from build123d import *

# Parameters (mm, degrees)
SKETCH_1_W                = 55
SKETCH_1_H                = 55
EXTRUDE_1_DEPTH           = 51
CUT_EXTRUDE_1_DEPTH       = 110.162722575
CHAMFER_1_SIZE            = 19.3
CUT_EXTRUDE_START         = -11
SKETCH_11_W               = 55
SKETCH_11_H               = 45
CUT_EXTRUDE_2_DEPTH       = 69.888985474
CUT_EXTRUDE_START_2       = 11
SKETCH_12_W               = 55
SKETCH_12_H               = 45
CUT_EXTRUDE_3_DEPTH       = 69.888985474
HOLE_WIZARD_M4_1_D        = 3.3
HOLE_WIZARD_M4_2_D        = 3.3
HOLE_WIZARD_1_D           = 6.6
HOLE_WIZARD_1_CBORE_D     = 11
HOLE_WIZARD_1_CBORE_DEPTH = 8
CUT_EXTRUDE_5_DEPTH       = 73.754724932
CUT_EXTRUDE_6_DEPTH       = 73.754724932
CHAMFER_2_SIZE            = 12
CUT_EXTRUDE_7_DEPTH       = 70.003623093


with BuildPart() as part:
    # 草图1 → 凸台-拉伸1 (new, symmetric)
    with BuildSketch(Plane.XY):
        Rectangle(SKETCH_1_W, SKETCH_1_H)
    extrude(amount=EXTRUDE_1_DEPTH, both=True)

    # 草图2 → 切除-拉伸1 (cut, through all)
    with BuildSketch(Plane.XY.offset(51)):
        Polygon((-27.5, -27.5), (16.5, -27.5), (-27.5, 16.5), align=None)
    extrude(amount=-CUT_EXTRUDE_1_DEPTH, mode=Mode.SUBTRACT)

    # 倒角1
    chamfer_1_edges = [part.edges().sort_by_distance(p)[0] for p in [
        (27.5, 27.5, 0),
    ]]
    chamfer(chamfer_1_edges, length=CHAMFER_1_SIZE)

    # 草图11 → 切除-拉伸2 (cut, through all)
    with BuildSketch(Plane.YZ.offset(27.5).offset(CUT_EXTRUDE_START)):
        with Locations((0, -28.5)):
            Rectangle(SKETCH_11_W, SKETCH_11_H)
    extrude(amount=-CUT_EXTRUDE_2_DEPTH, mode=Mode.SUBTRACT)

    # 草图12 → 切除-拉伸3 (cut, through all)
    with BuildSketch(Plane.XZ.offset(-27.5).offset(CUT_EXTRUDE_START_2)):
        with Locations((0, 28.5)):
            Rectangle(SKETCH_12_W, SKETCH_12_H)
    extrude(amount=CUT_EXTRUDE_3_DEPTH, mode=Mode.SUBTRACT)

    # M4 螺纹孔1 (through all)
    with Locations(Plane(origin=(16.5, -23.392318354, -4.126238011), x_dir=(0, 1, 0), z_dir=(-1, 0, 0))):
        with Locations((33.892318354, 26.873761989), (8.392318354, 41.596193853), (8.392318354, 12.151330125)):
            Hole(HOLE_WIZARD_M4_1_D / 2)

    # M4 螺纹孔2 (through all)
    with Locations(Plane(origin=(-3.776378322, 16.5, -11.360569787), x_dir=(-1, 0, 0), z_dir=(0, -1, 0))):
        with Locations((-14.276378322, -42.360569787), (11.223621678, -57.083001652), (11.223621678, -27.638137923)):
            Hole(HOLE_WIZARD_M4_2_D / 2)

    # 打孔尺寸根据内六角圆柱头螺钉的类型1 (through all)
    with Locations(Plane(origin=(-5.5, -5.5, 0), x_dir=(-0.7071067811865475, 0.7071067811865477, 0), z_dir=(-0.7071067811865477, -0.7071067811865475, 0))):
        with Locations((6.5, 0), (-6.5, 0)):
            CounterBoreHole(HOLE_WIZARD_1_D / 2, HOLE_WIZARD_1_CBORE_D / 2, HOLE_WIZARD_1_CBORE_DEPTH)

    # 草图22 → 切除-拉伸5 (cut, through all)
    with BuildSketch(Plane.XZ.offset(-16.5)):
        Polygon((3.2, 51), (15.2, 39), (15.2, 6), (19.2, 6), (19.2, 51), align=None)
    extrude(amount=-CUT_EXTRUDE_5_DEPTH, mode=Mode.SUBTRACT)

    # 草图23 → 切除-拉伸6 (cut, through all)
    with BuildSketch(Plane.ZY.offset(-16.5)):
        Polygon((-51, 19.2), (-51, 3.2), (-39, 15.2), (-6, 15.2), (-6, 19.2), align=None)
    extrude(amount=-CUT_EXTRUDE_6_DEPTH, mode=Mode.SUBTRACT)

    # 倒角2
    chamfer_2_edges = [part.edges().sort_by_distance(p)[0] for p in [
        (-27.5, 22, 51),
        (22, -27.5, -51),
    ]]
    chamfer(chamfer_2_edges, length=CHAMFER_2_SIZE)

    # 草图24 → 切除-拉伸7 (cut, through all)
    with BuildSketch(Plane(origin=(0, 0, -6), x_dir=(-1, 0, 0), z_dir=(0, 0, -1))):
        with BuildLine():
            Line((-5.122077939, 2.293650814), (-12.193145751, 9.364718626))
            ThreePointArc((-12.193145751, 9.364718626), (-12.193145751, 12.193145751), (-9.364718626, 12.193145751))
            Line((-9.364718626, 12.193145751), (-2.293650814, 5.122077939))
            ThreePointArc((-2.293650814, 5.122077939), (-2.293650814, 2.293650814), (-5.122077939, 2.293650814))
        make_face()
    extrude(amount=-CUT_EXTRUDE_7_DEPTH, mode=Mode.SUBTRACT)


solid = part.part
Read the model definition and answer for the solid it produces. Units are mm, in the model's axes. A direction names the side the tool comes from. Round coordinates to 2 decimals unless told otherwise and drop trailing zeros. Write each loop counter-clockwise with the first axis right and the second up, starting at its lowest first coordinate (ties: lowest second). Pieces come first, ordered by that corner, then holes.
1. The part is cut by section B-B, the plane x = -18.5. Determine the outline of the cut face in (y, z).
2. The part is cut by section A-A, the plane z = 31. Determine the outline of the cut face in (x, y), then the cut area to 3 significant figures.
3. Given pin 1 Ø4.5 at (x, z) = (-15, 45.72) entering from -Y; pin 2 Ø2 at (y, z) = (18, 21.5) entering from +X; pin 3 Ø3 at (x, z) = (0, 0) entering from -Y; pin 4 Ø3 at (y, z) = (-15, -45.72) entering from +X, each flat-ended and moving along its own axis, determine where each tip first touches the part or whether it passes through.
4. Straight lines are drawn through the part: L1, parallel to Z at x = 24.5, y = -15; L2, parallel to Z at x = -15, y = 21.5; L3, parallel to X at y = -25, z = -19. For each, find the intervals that lie inside material, in ascending order.
5. Which of the six approach directions +Z, -Z, +X, -X, +Y, -Y give full straight-line access (tool end or side, diameter ignored) to faces 4 (the face through (5.88, 8.71, -0.08)), 5 (the face through (2.215, -1.901, -0.077)), 6 (the face through (20.597, 8.926, -31.496))?
6. Determine the mould class of faces 1 (the face through (27.5, -10, -22)), 2 (the face through (21.9, -21.4, -45.1)), 3 (the face through (-6.46, 1.04, 5.37)) for opening direction Z: pulls with the +Z half, pulls with the -Z half, needs draft (parallel to the pull), parting line crosses it, or undercut.
Values:
1. outline: (7.5, -6) - (27.5, -6) - (27.5, 48) - (16.5, 48) - (16.5, 6) - (7.5, 6) - close
2. outline: (-27.5, 16.5) - (8.85, 16.5) - (8.85, 26.85) - (8.2, 27.5) - (-27.5, 27.5) - close; (12.15, 16.5) - (15.2, 16.5) - (15.2, 20.5) - (12.15, 23.55) - close
2. area: 416 mm2
3. pin 1: stops at y = 16.5
3. pin 2: stops at x = 15.2
3. pin 3: stops at y = -2.91
3. pin 4: passes through
4. L1: z = -51 to -47.37, -44.07 to -17.93, -14.63 to 6
4. L2: z = -6 to 14.63, 17.93 to 44.07, 47.37 to 51
4. L3: x = 16.5 to 27.5
5. face 4: +Z, -Z
5. face 5: none
5. face 6: +X, -X
6. face 1: needs draft
6. face 2: pulls with the -Z half
6. face 3: undercut
